CAD build for the part. Positions are in the model's coordinates, mm. A direction names the side the tool comes from. Round coordinates to 2 decimals unless told otherwise and drop trailing zeros. Loops run counter-clockwise (first coordinate to the right, second up) from the corner with the lowest first, then second, coordinate; pieces in that order, holes last.
from build123d import *

# Parameters (mm, degrees)
F0_W     = 12.446
F0_H     = 12.446
F0_R     = 4.572
F1_DEPTH = 25.4
F0_W_2   = 15.494
F0_H_2   = 15.494
F2_DEPTH = 2.54
F3_W     = 12.446
F3_H     = 12.446
F3_R     = 4.572
F4_DEPTH = 2.54
F5_R     = 2.54


with BuildPart() as f1:
    # F0 (on Top) → F1 (new body)
    with BuildSketch(Plane.XY):
        with Locations((6.223, 6.223)):
            Rectangle(F0_W, F0_H)
        with Locations((6.223, 6.223)):
            Circle(F0_R, mode=Mode.SUBTRACT)
    extrude(amount=F1_DEPTH)

    # F0 (on Top) → F2 (join)
    with BuildSketch(Plane.XY):
        with Locations((6.223, 6.223)):
            Rectangle(F0_W_2, F0_H_2)
        with Locations((6.223, 6.223)):
            Rectangle(F0_W, F0_H, mode=Mode.SUBTRACT)
    extrude(amount=F2_DEPTH)

    # F3 (on face) → F4 (join)
    with BuildSketch(Plane.XY.offset(25.4)):
        with Locations((6.223, 6.223)):
            Rectangle(F3_W, F3_H)
        with Locations((6.223, 6.223)):
            Circle(F3_R, mode=Mode.SUBTRACT)
        with Locations((6.223, 6.223)):
            Circle(F3_R)
    extrude(amount=F4_DEPTH)

    # F5
    f5_edges = [f1.edges().sort_by_distance(p)[0] for p in [
        (0, 12.446, 15.24),
        (12.446, 12.446, 15.24),
        (0, 0, 15.24),
        (12.446, 0, 15.24),
        (6.223, 12.446, 27.94),
        (12.446, 6.223, 27.94),
        (6.223, 0, 27.94),
        (0, 6.223, 27.94),
    ]]
    fillet(f5_edges, radius=F5_R)


solid = f1.part
Item 1: Cut at C-C (x = 9.5). List the corners of the cut face in (y, z), plus the area to 3 significant figures.
Verdict:
outline: (-1.52, 0) - (3.03, 0) - (3.03, 25.4) - (9.41, 25.4) - (9.41, 0) - (13.97, 0) - (13.97, 2.54) - (12.45, 2.54) - (12.45, 25.4) arc R2.54 ccw to (9.91, 27.94) - (2.54, 27.94) arc R2.54 ccw to (0, 25.4) - (0, 2.54) - (-1.52, 2.54) - close
area: 191 mm2
Item 2: Flat gauge pins, fed straight in: P1, Ø8, axis at y = 6.5, z = 13, coming from the -X side; P2, Ø1, axis at x = 12.5, z = 23.5, coming from the +Y side; P3, Ø6, axis at x = 7.5, z = 11, coming from the -Y side. Where does each tip first touch, or does it go through?
Verdict:
P1: stops at x = 0
P2: stops at y = 11.34
P3: stops at y = 0
Item 3: 3-axis set-ups, long thin cutter, end or side, ignore diameter. For faces 5 (the cylindrical face through (0.72, 11.68, 13.81)), 6 (the flat face through (6, 0, 14)), 7 (the flat face through (6, 12.446, 14)), 8 (the cylindrical face through (11.722, 11.682, 13.81)): which of +Z, -Z, +X, -X, +Y, -Y reach the whole face in a straight line?
Verdict:
face 5: +Z, -X, +Y
face 6: +Z, +X, -X, -Y
face 7: +Z, +X, -X, +Y
face 8: +Z, +X, +Y
Item 4: Cut at D-D (x = 0.5). List the corners of the cut face in (y, z).
Verdict:
outline: (-1.52, 0) - (13.97, 0) - (13.97, 2.54) - (11.42, 2.54) - (11.42, 25.4) arc R1.51 ccw to (9.91, 26.91) - (2.54, 26.91) arc R1.51 ccw to (1.03, 25.4) - (1.03, 2.54) - (-1.52, 2.54) - close
Item 5: Cut at B-B (y = 7.25). List the corners of the cut face in (x, z).
Verdict:
outline: (-1.52, 0) - (1.77, 0) - (1.77, 25.4) - (10.68, 25.4) - (10.68, 0) - (13.97, 0) - (13.97, 2.54) - (12.45, 2.54) - (12.45, 25.4) arc R2.54 ccw to (9.91, 27.94) - (2.54, 27.94) arc R2.54 ccw to (0, 25.4) - (0, 2.54) - (-1.52, 2.54) - close
Item 6: Mould opens along X. For faces 1 (the flat face through (10, 10, 0)), 2 (the flat face through (6, 6, 25.4)), 3 (the cylindrical face through (5.628, 10.756, 12.522)), 4 (the flat face through (12.446, 6, 14)) say: released by +X, released by -X, zero draft, split by the parting line, or undercut.
Verdict:
face 1: zero draft
face 2: undercut
face 3: undercut
face 4: released by +X
Item 7: Cut at A-A (z = 12). List the corners of the cut face in (x, y) (3 decimals).
Verdict:
outline: (0, 2.54) arc R2.54 ccw to (2.54, 0) - (9.906, 0) arc R2.54 ccw to (12.446, 2.54) - (12.446, 9.906) arc R2.54 ccw to (9.906, 12.446) - (2.54, 12.446) arc R2.54 ccw to (0, 9.906) - close; hole circle Ø9.144 at (6.223, 6.223)
Item 8: Wall check: L1, parallel to Z at x = 3, y = 9; L2, parallel to Z at x = 7, y = 12.5; L3, parallel to Y at x = 10, z = 19.25. Give the ranges that are in metal, low to high.
Verdict:
L1: z = 25.4 to 27.94
L2: z = 0 to 2.54
L3: y = 0 to 3.65, 8.8 to 12.44
